The listing builds one solid part. Answer for the finished solid, in the listing's coordinates (mm). A direction names the side the tool comes from. Give positions to 0.01 mm unless a question says otherwise; leave off trailing zeros. Loops run counter-clockwise (first coordinate to the right, second up) from the corner with the lowest first, then second, coordinate; pieces in that order, holes last.
Item 1: Section B-B, the plane x = 0 is taken. Give the vertices of the cut face in (y, z), and give its area (3 significant figures).
Item 2: Section D-D, the plane y = 37 is taken. Give the vertices of the cut face in (x, z).
Item 3: Section A-A, the plane y = 0 is taken. Give the vertices of the cut face in (x, z).
Item 4: Consider line 1 along Y through (x, z) = (-39, 0); line 2 along Y through (x, z) = (-1, 0); line 3 along Z through (x, y) = (4.5, -17). Determine where each line is inside the solid, lowest interval first.
Item 5: Each of these flat-tipped pins is pushed along its axis until it touches: pin 1 Ø1.6 at (y, z) = (36, 0) entering from -X; pin 2 Ø10 at (y, z) = (14.5, -6.5) entering from +X; pin 3 Ø1 at (y, z) = (2, -8.5) entering from +X; pin 4 Ø8 at (x, z) = (-31.5, -6.5) entering from +Y. Where does it stop, or does it pass through?
Item 6: A tool of negligible diameter and unlimited length cuts with its end or side. For faces 4 (the face through (-16.847, 25.04, 0.01)), 5 (the face through (-3, -13, 0)), 6 (the face through (-13.887, -10.648, -6.543)), from which of +Z, -Z, +X, -X, +Y, -Y can it reach the whole face along a straight path? Write none if from no direction.
Item 7: Section C-C, the plane z = 8 is taken. Give the vertices of the cut face in (x, y), and give its area (3 significant figures).
Item 8: The mould has two halves that part along Y. Classify faces 1 (the face through (25.04, 16.847, 0.01)), 2 (the face through (4, -11, -12.5)), 3 (the face through (12.42, -7.12, 0.18)): pulls with the +Y half, pulls with the -Y half, needs draft (parallel to the pull), parting line crosses it, or undercut.
from build123d import *

# Parameters (mm, degrees)
SKETCH1_R           = 17.5
SKETCH1_W           = 20
SKETCH1_H           = 15.1
SKETCH1_W_2         = 15.1
SKETCH1_H_2         = 20
BOSS_EXTRUDE1_DEPTH = 0.75
SKETCH1_3_R         = 17.5
BOSS_EXTRUDE2_DEPTH = 12.5


with BuildPart() as part:
    # Sketch1 → Boss-Extrude1 (new, symmetric)
    with BuildSketch(Plane.XY):
        with BuildLine():
            Line((-6, -57.5), (6, -57.5))
            ThreePointArc((6, -57.5), (13.071067812, -54.571067812), (16, -47.5))
            Line((16, -47.5), (16, -29.068883707))
            ThreePointArc((16, -29.068883707), (16.871290708, -24.986400803), (19.333333333, -21.615323782))
            ThreePointArc((19.333333333, -21.615323782), (20.506096654, -20.506096654), (21.615323782, -19.333333333))
            ThreePointArc((21.615323782, -19.333333333), (24.986400803, -16.871290708), (29.068883707, -16))
            Line((29.068883707, -16), (47.5, -16))
            ThreePointArc((47.5, -16), (54.571067812, -13.071067812), (57.5, -6))
            Line((57.5, -6), (57.5, 6))
            ThreePointArc((57.5, 6), (54.571067812, 13.071067812), (47.5, 16))
            Line((47.5, 16), (29.068883707, 16))
            ThreePointArc((29.068883707, 16), (24.986400803, 16.871290708), (21.615323782, 19.333333333))
            ThreePointArc((21.615323782, 19.333333333), (20.506096654, 20.506096654), (19.333333333, 21.615323782))
            ThreePointArc((19.333333333, 21.615323782), (16.871290708, 24.986400803), (16, 29.068883707))
            Line((16, 29.068883707), (16, 47.5))
            ThreePointArc((16, 47.5), (13.071067812, 54.571067812), (6, 57.5))
            Line((6, 57.5), (-6, 57.5))
            ThreePointArc((-6, 57.5), (-13.071067812, 54.571067812), (-16, 47.5))
            Line((-16, 47.5), (-16, 29.068883707))
            ThreePointArc((-16, 29.068883707), (-16.871290708, 24.986400803), (-19.333333333, 21.615323782))
            ThreePointArc((-19.333333333, 21.615323782), (-20.506096654, 20.506096654), (-21.615323782, 19.333333333))
            ThreePointArc((-21.615323782, 19.333333333), (-24.986400803, 16.871290708), (-29.068883707, 16))
            Line((-29.068883707, 16), (-47.5, 16))
            ThreePointArc((-47.5, 16), (-54.571067812, 13.071067812), (-57.5, 6))
            Line((-57.5, 6), (-57.5, -6))
            ThreePointArc((-57.5, -6), (-54.571067812, -13.071067812), (-47.5, -16))
            Line((-47.5, -16), (-29.068883707, -16))
            ThreePointArc((-29.068883707, -16), (-24.986400803, -16.871290708), (-21.615323782, -19.333333333))
            ThreePointArc((-21.615323782, -19.333333333), (-20.506096654, -20.506096654), (-19.333333333, -21.615323782))
            ThreePointArc((-19.333333333, -21.615323782), (-16.871290708, -24.986400803), (-16, -29.068883707))
            Line((-16, -29.068883707), (-16, -47.5))
            ThreePointArc((-16, -47.5), (-13.071067812, -54.571067812), (-6, -57.5))
        make_face()
        Circle(SKETCH1_R, mode=Mode.SUBTRACT)
        with Locations((0, 35)):
            Rectangle(SKETCH1_W, SKETCH1_H, mode=Mode.SUBTRACT)
        with Locations((0, -35)):
            Rectangle(SKETCH1_W, SKETCH1_H, mode=Mode.SUBTRACT)
        with Locations((35, 0)):
            Rectangle(SKETCH1_W_2, SKETCH1_H_2, mode=Mode.SUBTRACT)
        with Locations((-35, 0)):
            Rectangle(SKETCH1_W_2, SKETCH1_H_2, mode=Mode.SUBTRACT)
    extrude(amount=BOSS_EXTRUDE1_DEPTH, both=True)

    # Sketch1<3> → Boss-Extrude2 (add, symmetric)
    with BuildSketch(Plane.XY):
        Circle(SKETCH1_3_R)
        with BuildLine():
            ThreePointArc((-8.114442262, 8.148977039), (-5.75, 9.959292144), (-3, 11.101801656))
            Line((-3, 11.101801656), (-3, 14))
            ThreePointArc((-3, 14), (0, 14.317821063), (3, 14))
            Line((3, 14), (3, 11.101801656))
            ThreePointArc((3, 11.101801656), (5.75, 9.959292144), (8.114442262, 8.148977039))
            Line((8.114442262, 8.148977039), (10.624355653, 9.598076211))
            ThreePointArc((10.624355653, 9.598076211), (12.399596768, 7.158910532), (13.624355653, 4.401923789))
            Line((13.624355653, 4.401923789), (11.114442262, 2.952824616))
            ThreePointArc((11.114442262, 2.952824616), (11.5, 0), (11.114442262, -2.952824616))
            Line((11.114442262, -2.952824616), (13.624355653, -4.401923789))
            ThreePointArc((13.624355653, -4.401923789), (12.399596768, -7.158910532), (10.624355653, -9.598076211))
            Line((10.624355653, -9.598076211), (8.114442262, -8.148977039))
            ThreePointArc((8.114442262, -8.148977039), (5.75, -9.959292144), (3, -11.101801656))
            Line((3, -11.101801656), (3, -14))
            ThreePointArc((3, -14), (0, -14.317821063), (-3, -14))
            Line((-3, -14), (-3, -11.101801656))
            ThreePointArc((-3, -11.101801656), (-5.75, -9.959292144), (-8.114442262, -8.148977039))
            Line((-8.114442262, -8.148977039), (-10.624355653, -9.598076211))
            ThreePointArc((-10.624355653, -9.598076211), (-12.399596768, -7.158910532), (-13.624355653, -4.401923789))
            Line((-13.624355653, -4.401923789), (-11.114442262, -2.952824616))
            ThreePointArc((-11.114442262, -2.952824616), (-11.5, 0), (-11.114442262, 2.952824616))
            Line((-11.114442262, 2.952824616), (-13.624355653, 4.401923789))
            ThreePointArc((-13.624355653, 4.401923789), (-12.399596768, 7.158910532), (-10.624355653, 9.598076211))
            Line((-10.624355653, 9.598076211), (-8.114442262, 8.148977039))
        make_face(mode=Mode.SUBTRACT)
    extrude(amount=BOSS_EXTRUDE2_DEPTH, both=True)


solid = part.part
Worked answers:
1. outline: (-57.5, -0.75) - (-42.55, -0.75) - (-42.55, 0.75) - (-57.5, 0.75) - close; (-27.45, -0.75) - (-17.5, -0.75) - (-17.5, -12.5) - (-14.32, -12.5) - (-14.32, 12.5) - (-17.5, 12.5) - (-17.5, 0.75) - (-27.45, 0.75) - close; (14.32, -12.5) - (17.5, -12.5) - (17.5, -0.75) - (27.45, -0.75) - (27.45, 0.75) - (17.5, 0.75) - (17.5, 12.5) - (14.32, 12.5) - close; (42.55, -0.75) - (57.5, -0.75) - (57.5, 0.75) - (42.55, 0.75) - close
1. area: 234 mm2
2. outline: (-16, -0.75) - (-10, -0.75) - (-10, 0.75) - (-16, 0.75) - close; (10, -0.75) - (16, -0.75) - (16, 0.75) - (10, 0.75) - close
3. outline: (-57.5, -0.75) - (-42.55, -0.75) - (-42.55, 0.75) - (-57.5, 0.75) - close; (-27.45, -0.75) - (-17.5, -0.75) - (-17.5, -12.5) - (-11.5, -12.5) - (-11.5, 12.5) - (-17.5, 12.5) - (-17.5, 0.75) - (-27.45, 0.75) - close; (11.5, -12.5) - (17.5, -12.5) - (17.5, -0.75) - (27.45, -0.75) - (27.45, 0.75) - (17.5, 0.75) - (17.5, 12.5) - (11.5, 12.5) - close; (42.55, -0.75) - (57.5, -0.75) - (57.5, 0.75) - (42.55, 0.75) - close
4. line 1: y = -16 to -10, 10 to 16
4. line 2: y = -57.5 to -42.55, -27.45 to -14.28, 14.28 to 27.45, 42.55 to 57.5
4. line 3: z = -0.75 to 0.75
5. pin 1: stops at x = -16
5. pin 2: stops at x = 14.7
5. pin 3: stops at x = 17.44
5. pin 4: passes through
6. face 4: +Z, -Z, -X, +Y
6. face 5: +Z, -Z
6. face 6: -Z
7. outline: circle Ø35 at (0, 0); hole (-13.62, -4.4) arc R14.32 ccw to (-10.62, -9.6) - (-8.11, -8.15) arc R11.5 ccw to (-3, -11.1) - (-3, -14) arc R14.32 ccw to (3, -14) - (3, -11.1) arc R11.5 ccw to (8.11, -8.15) - (10.62, -9.6) arc R14.32 ccw to (13.62, -4.4) - (11.11, -2.95) arc R11.5 ccw to (11.11, 2.95) - (13.62, 4.4) arc R14.32 ccw to (10.62, 9.6) - (8.11, 8.15) arc R11.5 ccw to (3, 11.1) - (3, 14) arc R14.32 ccw to (-3, 14) - (-3, 11.1) arc R11.5 ccw to (-8.11, 8.15) - (-10.62, 9.6) arc R14.32 ccw to (-13.62, 4.4) - (-11.11, 2.95) arc R11.5 ccw to (-11.11, -2.95) - close
7. area: 444 mm2
8. face 1: pulls with the +Y half
8. face 2: needs draft
8. face 3: undercut
